CAD build for the part. Positions are in the model's coordinates, mm. Face numbers are marked on the shaded views. A direction names the side the tool comes from. Coordinates: 2 decimals unless noted, no trailing zeros. Loops run counter-clockwise (first coordinate to the right, second up) from the corner with the lowest first, then second, coordinate; pieces in that order, holes last. Notation, with made-up numbers: (7.5, 10) -> (65.5, 10) arc R25 cw to (65.5, 28) -> close; hole circle Ø11 at (79, -16.75). An arc over 180 degrees is marked (long way). Return JSON: item names as keys, results as strings. Group by question number.
(1) Saw through at A-A on y = -3.75. Write the cut outline in (x, z).
(2) Flat gauge pins, fed straight in: pin 1 Ø1.6 at (y, z) = (-3.5, 0) entering from -X; pin 2 Ø1.5 at (x, y) = (1, -2) entering from -Z; pin 3 Ø1.6 at (y, z) = (-3.5, 0) entering from +X. Where does each tip first touch, or does it go through?
(3) Mould opens along Z. For the marked faces 3, 4 and 5 say: pulls with the +Z half, pulls with the -Z half, needs draft (parallel to the pull), parting line crosses it, or undercut.
(4) Tool access for the marked faces 1 and 2: list every direction of +Z, -Z, +X, -X, +Y, -Y with a clear straight run to the whole face (end or side of a thin tool).
(5) Probe L1, parallel to Z at x = 0, y = -0.5; L2, parallel to X at y = -4, z = 0.75; L3, parallel to Y at x = 1.5, z = 2.25. List the from-to ranges inside material, lowest first.
```python
from build123d import *

# Parameters (mm, degrees)
SKETCH3_R           = 2.55
BOSS_EXTRUDE1_DEPTH = 5
SKETCH4_W           = 3.1
SKETCH4_H           = 3.1
CUT_EXTRUDE1_DEPTH  = 2


with BuildPart() as part:
    # Sketch1 → Revolve5 (revolve)
    with BuildSketch(Plane(origin=(0, 0, 0), x_dir=(0, 0, -1), z_dir=(1, 0, 0))):
        with BuildLine():
            Line((0, 3), (0, 0))
            Line((0, 0), (3.5, 0))
            add(Edge.make_bspline(
                [(3.5, 0), (3.5, 3), (0, 3)],
                knots=[3.141592654, 3.141592654, 3.141592654, 4.71238898, 4.71238898, 4.71238898], degree=2, weights=[1, 0.707106781, 1]))
        make_face()
    revolve(axis=Axis((0, 0, 0), (0, 1, 0)))

    # Sketch3 → Boss-Extrude1 (add)
    with BuildSketch(Plane.XZ):
        Circle(SKETCH3_R)
    extrude(amount=BOSS_EXTRUDE1_DEPTH)

    # Sketch4 → Cut-Extrude1 (cut)
    with BuildSketch(Plane.XZ.offset(5)):
        Rectangle(SKETCH4_W, SKETCH4_H)
    extrude(amount=-CUT_EXTRUDE1_DEPTH, mode=Mode.SUBTRACT)


solid = part.part
```
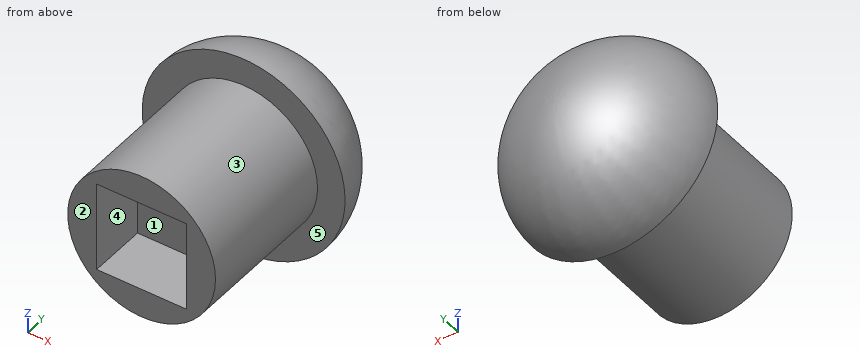
Geometry results:
{
 "1": {"outline": "circle Ø5.1 at (0, 0); hole (-1.55, -1.55) -> (1.55, -1.55) -> (1.55, 1.55) -> (-1.55, 1.55) -> close"},
 "2": {"pin 1": "x = -2.55", "pin 2": "z = -2.54", "pin 3": "x = 2.55"},
 "3": {"face 3": "parting line crosses it", "face 4": "undercut", "face 5": "needs draft"},
 "4": {"face 1": "-Y", "face 2": "+Z, -Z, +X, -X, -Y"},
 "5": {"L1": "-2.55 to 2.55", "L2": "-2.44 to -1.55, 1.55 to 2.44", "L3": "0 to 1.9"}
}
